from build123d import *

# Parameters (mm, degrees)
F0_R     = 152.4
F1_DEPTH = 635
F3_DEPTH = 317.5
F4_R     = 127


with BuildPart() as f1:
    # F0 (on Top) → F1 (new body)
    with BuildSketch(Plane.XY):
        with BuildLine():
            ThreePointArc((243.959033, -203.2), (298.549195, -108.049195), (317.5, 0))
            ThreePointArc((317.5, 0), (298.549195, 108.049195), (243.959033, 203.2))
            ThreePointArc((243.959033, 203.2), (-317.5, 0), (243.959033, -203.2))
        make_face()
        Circle(F0_R, mode=Mode.SUBTRACT)
        with BuildLine():
            ThreePointArc((243.959033, 203.2), (298.549195, 108.049195), (317.5, 0))
            ThreePointArc((317.5, 0), (298.549195, -108.049195), (243.959033, -203.2))
            Line((243.959033, -203.2), (2006.6, -203.2))
            ThreePointArc((2006.6, -203.2), (1905, 0), (2006.6, 203.2))
            Line((2006.6, 203.2), (243.959033, 203.2))
        make_face()
        with BuildLine():
            ThreePointArc((2413, 0), (2272.592253, 227.184507), (2006.6, 203.2))
            ThreePointArc((2006.6, 203.2), (1905, 0), (2006.6, -203.2))
            ThreePointArc((2006.6, -203.2), (2272.592253, -227.184507), (2413, 0))
        make_face()
        with Locations((2159, 0)):
            Circle(F0_R, mode=Mode.SUBTRACT)
    extrude(amount=F1_DEPTH)

    # F2 (on Front) → F3 (intersect, symmetric)
    with BuildSketch(Plane.XZ):
        Polygon((-317.5, 203.2), (-317.5, 0), (508, 0), (1804.455024, 228.6), (2413, 228.6), (2413, 431.8), (1786.677328, 431.8), (490.222304, 203.2), align=None)
    extrude(amount=F3_DEPTH, both=True, mode=Mode.INTERSECT)

    # F4
    f4_edges = [f1.edges().sort_by_distance(p)[0] for p in [
        (2006.6, 203.2, 330.2),
        (243.959033, 203.2, 101.6),
        (243.959033, -203.2, 101.6),
        (2006.6, -203.2, 330.2),
    ]]
    fillet(f4_edges, radius=F4_R)


solid = f1.part
Build history of the part. All positions in model axes, mm. A direction names the side the tool comes from. Give positions to 0.01 mm unless a question says otherwise; leave off trailing zeros. Loops run counter-clockwise (first coordinate to the right, second up) from the corner with the lowest first, then second, coordinate; pieces in that order, holes last. Notation, with made-up numbers: (61, 41) - (84, 41) arc R14 ccw to (84, 45) - close; hole circle Ø11 at (6.5, 71.25). An arc over 180 degrees is marked (long way). Write item = value, one per line. Start each with the question number.
1) Band-saw the part on D-D on x = 2159. Give the cut face in (y, z).
2) Drop flat-ended pins along their axis: pin 1 Ø1.5 at (y, z) = (133, 119) entering from -X; pin 2 Ø3 at (y, z) = (-149, 93) entering from -X; pin 3 Ø1 at (x, z) = (1588, 308) entering from +Y. Give the stop position or say it passes through.
3) Band-saw the part on A-A on x = 0. Give the cut face in (y, z).
4) Pull direction Y, two halves, no side cores. Call faces 5 (the flat face through (1147.15, -2.84, 112.7)), 6 (the flat face through (1145, 203.2, 213)), 7 (the cylindrical face through (-120.94, -92.73, 100.18)): +Y half, -Y half, draft (parallel to the pull), parting line (faces both ways), or undercut.
5) Band-saw the part on B-B on y = 113.5. Give the cut face in (x, z), plus the area to 3 significant figures.
6) Band-saw the part on C-C on z = 324.5. Give the cut face in (x, y).
7) Probe probe 1 along Y at (x, z) = (0, 136); probe 2 along Y at (x, z) = (2159, 298); probe 3 along Z at (x, y) = (142, 259.5). List the from-to ranges inside material, lowest first. Write a range as from..to.
8) Tool access for faces 1 (the flat face through (182, -4, 203.2)), 2 (the flat face through (1122, -203.2, 213)), 3 (the flat face through (1969, -4, 228.6)), 4 (the cylindrical face through (2001.27, -207.39, 331.62)): list every direction of +Z, -Z, +X, -X, +Y, -Y with a clear straight run to the whole face (end or side of a thin tool).
Final values:
q1.outline = (-254, 228.6) - (-152.4, 228.6) - (-152.4, 431.8) - (-254, 431.8) - close; (152.4, 228.6) - (254, 228.6) - (254, 431.8) - (152.4, 431.8) - close
q2.pin_1 = -288.65
q2.pin_2 = -281.16
q2.pin_3 = 203.2
q3.outline = (-317.5, 0) - (-152.4, 0) - (-152.4, 203.2) - (-317.5, 203.2) - close; (152.4, 0) - (317.5, 0) - (317.5, 203.2) - (152.4, 203.2) - close
q4.face_5 = draft
q4.face_6 = +Y half
q4.face_7 = undercut
q5.outline = (-296.52, 0) - (-101.7, 0) - (-101.7, 203.2) - (-296.52, 203.2) - close; (101.7, 0) - (508, 0) - (1804.46, 228.6) - (2057.3, 228.6) - (2057.3, 431.8) - (1786.68, 431.8) - (490.22, 203.2) - (101.7, 203.2) - close; (2260.7, 228.6) - (2386.23, 228.6) - (2386.23, 431.8) - (2260.7, 431.8) - close
q5.area = 467,000 mm²
q6.outline = (1178.15, -203.2) - (1968.92, -203.2) arc R127 cw to (2032.28, -220.13) arc R254 ccw to (2413, 0) arc R254 ccw to (2032.28, 220.13) arc R127 cw to (1968.92, 203.2) - (1178.15, 203.2) - close; hole circle Ø304.8 at (2159, 0)
q7.probe_1 = -317.5..-152.4, 152.4..317.5
q7.probe_2 = -254..-152.4, 152.4..254
q7.probe_3 = 0..203.2
q8.face_1 = +Z, -X, +Y, -Y
q8.face_2 = +Z, -Z, -Y
q8.face_3 = -Z, +X, +Y, -Y
q8.face_4 = +Z, -Z, -X, -Y
